from build123d import *

# Parameters (mm, degrees)
AXLE_BASE_SKETCH_R        = 19
AXLE_DEPTH                = 98.5
GUARD_BASE_R              = 30
GUARD_DEPTH               = 5
INNER_AXLE_HOLE_BASE_R    = 8.5
INNER_AXLE_HOLE_DEPTH     = 104.5
BEND_ROOM_BASE_W          = 1.5
BEND_ROOM_BASE_H          = 50
BEND_ROOM_1_DEPTH         = 66
BEND_ROOM_2_COUNT         = 2
BEND_ROOM_2_ANGLE         = 90
EASY_REMOVAL_CHAMFER_SIZE = 4


with BuildPart() as part:
    # Axle base sketch → Axle (new body)
    with BuildSketch(Plane.XY):
        Circle(AXLE_BASE_SKETCH_R)
    extrude(amount=AXLE_DEPTH)

    # Guard base → Guard (add)
    with BuildSketch(Plane(origin=(0, 0, 0), x_dir=(-1, 0, 0), z_dir=(0, 0, -1))):
        Circle(GUARD_BASE_R)
    extrude(amount=GUARD_DEPTH)

    # Inner axle hole base → Inner axle hole (cut, through all)
    with BuildSketch(Plane.XY.offset(98.5)):
        Circle(INNER_AXLE_HOLE_BASE_R)
    extrude(amount=-INNER_AXLE_HOLE_DEPTH, mode=Mode.SUBTRACT)

    # Mate ring base → Mate rings (revolve)
    with BuildSketch(Plane(origin=(0, 0, 0), x_dir=(1, 0, 0), z_dir=(0, 1, 0))):
        Polygon((19, -98.5), (19.75, -97.75), (19.75, -97), (19, -96.25), align=None)
        Polygon((19, -92.75), (19.75, -92), (19.75, -91.25), (19, -90.5), align=None)
    revolve(axis=Axis((0, 0, 0), (0, 0, -1)))

    # Bend room base → Bend room 1 (cut)
    with BuildSketch(Plane.XY.offset(98.5)):
        Rectangle(BEND_ROOM_BASE_W, BEND_ROOM_BASE_H)
    bend_room_1 = extrude(amount=-BEND_ROOM_1_DEPTH, mode=Mode.SUBTRACT)

    # Bend room 2: Bend room 1 ×2 about axis
    bend_room_2_axis = Axis((0, 0, 0), (0, 0, -1))
    for i in range(1, BEND_ROOM_2_COUNT):
        add(bend_room_1.rotate(bend_room_2_axis, i * BEND_ROOM_2_ANGLE / (BEND_ROOM_2_COUNT - 1)), mode=Mode.SUBTRACT)

    # Easy removal chamfer
    easy_removal_chamfer_edges = [part.edges().sort_by_distance(p)[0] for p in [
        (30, 0, 0),
    ]]
    chamfer(easy_removal_chamfer_edges, length=EASY_REMOVAL_CHAMFER_SIZE)


solid = part.part
Verification items for the finished model (mm, model axes). A direction names the side the tool comes from. Coordinates: 2 decimals unless noted, no trailing zeros. Loops run counter-clockwise (first coordinate to the right, second up) from the corner with the lowest first, then second, coordinate; pieces in that order, holes last. Notation, with made-up numbers: M 77.25,-34.75 L 86.25,-34.75 A16 ccw 86.25,-6.75 Z; hole C 9,23 d6. An arc over 180 degrees is marked long. One line per item, written item: value.
1. Material ranges on line 1 along X through (y, z) = (-17, 34); line 2 along Z through (x, y) = (21.5, 2); line 3 along Y through (x, z) = (0, 30), recorded low to high. Write a range as from..to.
Answers follow:
line 1: -8.49..-0.75, 0.75..8.49
line 2: -5..0
line 3: -19..-8.5, 8.5..19
2. Section check A-A on z = 54.5. Record the cut outline in (x, y), plus the area to 3 significant figures.
Answers follow:
outline: M -18.99,-0.75 A19 ccw -0.75,-18.99 L -0.75,-8.47 A8.5 cw -8.47,-0.75 Z; M -18.99,0.75 L -8.47,0.75 A8.5 cw -0.75,8.47 L -0.75,18.99 A19 ccw Z; M 0.75,-18.99 A19 ccw 18.99,-0.75 L 8.47,-0.75 A8.5 cw 0.75,-8.47 Z; M 0.75,8.47 A8.5 cw 8.47,0.75 L 18.99,0.75 A19 ccw 0.75,18.99 Z
area: 844 mm^2
3. Set-up check for faces 1 (the conical face through (-13.38, -13.66, 90.62)), 2 (the cylindrical face through (13.82, 14.11, 97.37)), 3 (the flat face through (14, 0.75, 66)), 4 (the conical face through (13.66, -13.38, 96.37)), 5 (the flat face through (-0.75, 14, 66)): record each of +Z, -Z, +X, -X, +Y, -Y from which the full face is reachable in a straight line by a thin tool's end or side.
Answers follow:
face 1: -X, -Y
face 2: +Z, +X, +Y
face 3: +Z, +X, -X
face 4: +X, -Y
face 5: +Z, +Y, -Y
4. Gauge pin test, flat ends, axial feed: P1, Ø9, axis at y = -13.5, z = 78.5, coming from the +X side; P2, Ø5.5, axis at x = 14.5, z = 69.5, coming from the +Y side; P3, Ø3, axis at y = 11.5, z = 60.5, coming from the -X side. Record the tip position at first contact, or that the pin passes through.
Answers follow:
P1: x = 16.73
P2: y = 14.93
P3: x = -16.16
5. Section check B-B on z = 14.5. Record the cut outline in (x, y), plus the area to 3 significant figures.
Answers follow:
outline: C 0,0 d38; hole C 0,0 d17
area: 907 mm^2
6. Mould release check, pull along X, two halves, no side actions. Record for faces 6 (the conical face through (13.38, 13.67, 92.62)), 7 (the flat face through (-14, 0.75, 66)), 8 (the flat face through (-0.75, -13, 66)): pulls with the +X half, pulls with the -X half, needs draft (parallel to the pull), parting line crosses it, or undercut.
Answers follow:
face 6: pulls with the +X half
face 7: needs draft
face 8: undercut
